```python
from build123d import *

# Parameters (mm, degrees)
SKETCH1_W           = 21
SKETCH1_H           = 19
BOSS_EXTRUDE2_DEPTH = 10
SKETCH3_W           = 16.2
SKETCH3_H           = 14.2
CUT_EXTRUDE1_DEPTH  = 2.019279387
SKETCH4_R           = 1
CUT_EXTRUDE2_DEPTH  = 8


with BuildPart() as part:
    # Sketch1 → Boss-Extrude2 (new body)
    with BuildSketch(Plane.XY):
        Rectangle(SKETCH1_W, SKETCH1_H)
    extrude(amount=BOSS_EXTRUDE2_DEPTH)

    # Sketch3 → Cut-Extrude1 (cut)
    with BuildSketch(Plane(origin=(0, 0, 0), x_dir=(-1, 0, 0), z_dir=(0, 0, -1))):
        Rectangle(SKETCH3_W, SKETCH3_H)
    extrude(amount=-CUT_EXTRUDE1_DEPTH, mode=Mode.SUBTRACT)

    # Sketch4 → Cut-Extrude2 (cut)
    with BuildSketch(Plane(origin=(0, 0, 2.019279387), x_dir=(-1, 0, 0), z_dir=(0, 0, -1))):
        Circle(SKETCH4_R)
    extrude(amount=-CUT_EXTRUDE2_DEPTH, mode=Mode.SUBTRACT)


solid = part.part
```
Geometry check sheet. Reference: the model listing, model coordinates, mm. A direction names the side the tool comes from. Round coordinates to 2 decimals unless told otherwise and drop trailing zeros. Loops run counter-clockwise (first coordinate to the right, second up) from the corner with the lowest first, then second, coordinate; pieces in that order, holes last. Notation, with made-up numbers: (58, -15) - (112, -15) arc R13 cw to (112, 7) - close; hole circle Ø1 at (-5, 49.5). An arc over 180 degrees is marked (long way). Use a Markdown table: item, result.
Q1. Draft check along X on faces 3 (the flat face through (0, -9.5, 5)), 4 (the flat face through (-10.5, 0, 5)), 5 (the flat face through (0, -7.1, 1)). Enter one of: released by +X, released by -X, zero draft, split by the parting line, or undercut.
Solutions:
| item | result |
|---|---|
| face 3 | zero draft |
| face 4 | released by -X |
| face 5 | undercut |
Q2. Cross-section at C-C on y = 0. Record the cut outline in (x, z).
Solutions:
| item | result |
|---|---|
| outline | (-10.5, 0) - (-8.1, 0) - (-8.1, 2.02) - (-1, 2.02) - (-1, 10) - (-10.5, 10) - close; (1, 2.02) - (8.1, 2.02) - (8.1, 0) - (10.5, 0) - (10.5, 10) - (1, 10) - close |
Q3. Go/stop test with a flat-tipped pin: P1, Ø2.5, axis at x = 0, y = 0, coming from the -Z side. Record where the tip stops, or that it passes through.
Solutions:
| item | result |
|---|---|
| P1 | stops at z = 2.02 |
Q4. Access from +Z, -Z, +X, -X, +Y, -Y to the whole of each face (thin tool, end or side, straight path). Record for faces 1 (the flat face through (0, 2, 2.019)), 2 (the flat face through (0, 2, 10)).
Solutions:
| item | result |
|---|---|
| face 1 | -Z |
| face 2 | +Z, +X, -X, +Y, -Y |
Q5. Material ranges on line 1 (Y direction, x = 0, z = 7.25); line 2 (Z direction, x = 7.5, y = -7); line 3 (X direction, y = 2, z = 1.5), recorded low to high.
Solutions:
| item | result |
|---|---|
| line 1 | y = -9.5 to -1, 1 to 9.5 |
| line 2 | z = 2.02 to 10 |
| line 3 | x = -10.5 to -8.1, 8.1 to 10.5 |
Q6. Cross-section at B-B on y = -5.25. Record the cut outline in (x, z), plus the area to 3 significant figures.
Solutions:
| item | result |
|---|---|
| outline | (-10.5, 0) - (-8.1, 0) - (-8.1, 2.02) - (8.1, 2.02) - (8.1, 0) - (10.5, 0) - (10.5, 10) - (-10.5, 10) - close |
| area | 177 mm2 |
Q7. Cross-section at D-D on z = 1.25. Record the cut outline in (x, y).
Solutions:
| item | result |
|---|---|
| outline | (-10.5, -9.5) - (10.5, -9.5) - (10.5, 9.5) - (-10.5, 9.5) - close; hole (-8.1, -7.1) - (8.1, -7.1) - (8.1, 7.1) - (-8.1, 7.1) - close |
Q8. Cross-section at A-A on x = 0. Record the cut outline in (y, z), plus the area to 3 significant figures.
Solutions:
| item | result |
|---|---|
| outline | (-9.5, 0) - (-7.1, 0) - (-7.1, 2.02) - (-1, 2.02) - (-1, 10) - (-9.5, 10) - close; (1, 2.02) - (7.1, 2.02) - (7.1, 0) - (9.5, 0) - (9.5, 10) - (1, 10) - close |
| area | 145 mm2 |
